```python
from build123d import *

# Parameters (mm, degrees)
SKETCH_1_W             = 220
SKETCH_1_H             = 5.5
EXTRUDE_1_DEPTH        = 5
EXTRUDE_2_DEPTH        = 5
PATTERN_LINEAR_1_COUNT = 35
PATTERN_LINEAR_1_PITCH = 6.283185307
SKETCH_4_W             = 16.5
SKETCH_4_H             = 38
SKETCH_4_R             = 1.25
SKETCH_4_W_2           = 12.5
SKETCH_4_H_2           = 23.5
EXTRUDE_1_2_DEPTH      = 22
SKETCH_5_W             = 12.5
SKETCH_5_H             = 34
CUT_EXTRUDE_1_DEPTH    = 20
SKETCH_6_W             = 9
SKETCH_6_H             = 8
CUT_EXTRUDE_2_DEPTH    = 225.290548174


with BuildPart() as part:
    # 草图1 → Extrude 1 (new body)
    with BuildSketch(Plane.XY):
        with Locations((110, -2.75)):
            Rectangle(SKETCH_1_W, SKETCH_1_H)
    extrude(amount=EXTRUDE_1_DEPTH)

    # 草图2 → 拉伸2 (add)
    with BuildSketch(Plane.XY.offset(5)):
        Polygon((0, 0), (1.637866054, 4.5), (3.323577771, 4.5), (4.961443825, 0), align=None)
    extrude_2 = extrude(amount=-EXTRUDE_2_DEPTH)

    # 阵列(线性)1: 拉伸2 ×35
    with Locations(*[(i * PATTERN_LINEAR_1_PITCH, 0, 0) for i in range(1, PATTERN_LINEAR_1_COUNT)]):
        add(extrude_2)

    # 草图4 → Extrude 1 2 (add)
    with BuildSketch(Plane(origin=(220, 0, 0), x_dir=(0, 0, -1), z_dir=(1, 0, 0))):
        with Locations((-13.25, 13.5)):
            Rectangle(SKETCH_4_W, SKETCH_4_H)
        with Locations((-16.75, 27.5)):
            Circle(SKETCH_4_R, mode=Mode.SUBTRACT)
        with Locations(Location((-9.75, 27.5, 0), (0, 0, 180))):
            Circle(SKETCH_4_R, mode=Mode.SUBTRACT)
        with Locations((-9.75, -0.5)):
            Circle(SKETCH_4_R, mode=Mode.SUBTRACT)
        with Locations(Location((-16.75, -0.5, 0), (0, 0, 180))):
            Circle(SKETCH_4_R, mode=Mode.SUBTRACT)
        with Locations((-13.25, 13.5)):
            Rectangle(SKETCH_4_W_2, SKETCH_4_H_2, mode=Mode.SUBTRACT)
    extrude(amount=-EXTRUDE_1_2_DEPTH)

    # 草图5 → 切除-拉伸1 (cut)
    with BuildSketch(Plane.ZY.offset(-198)):
        with Locations((13.25, 13.5)):
            Rectangle(SKETCH_5_W, SKETCH_5_H)
    extrude(amount=-CUT_EXTRUDE_1_DEPTH, mode=Mode.SUBTRACT)

    # 草图6 → 切除-拉伸2 (cut, through all)
    with BuildSketch(Plane(origin=(0, 32.5, 0), x_dir=(1, 0, 0), z_dir=(0, 1, 0))):
        with Locations((202.5, -13.25)):
            Rectangle(SKETCH_6_W, SKETCH_6_H)
    extrude(amount=-CUT_EXTRUDE_2_DEPTH, mode=Mode.SUBTRACT)


solid = part.part
```
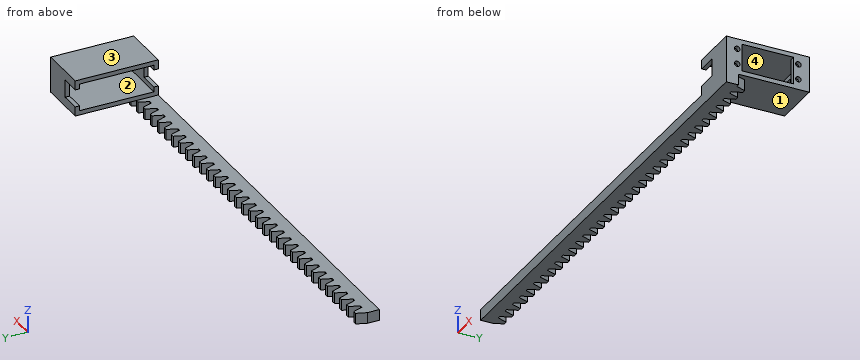
Part model, mm, in its own coordinate system. Face numbers are marked on the shaded views. A direction names the side the tool comes from. Round coordinates to 2 decimals unless told otherwise and drop trailing zeros. Loops run counter-clockwise (first coordinate to the right, second up) from the corner with the lowest first, then second, coordinate; pieces in that order, holes last. Notation, with made-up numbers: (-6, 18) -> (25, 18) arc R22 cw to (25, 26) -> close; hole circle Ø3 at (80.5, 29.25). An arc over 180 degrees is marked (long way). Use one line per item in the form item = value. Start each with the question number.
Item 1: Drill centre lines: line 1 along Y through (x, z) = (218.7, 9.75); line 2 along Z through (x, y) = (209, 21); line 3 along Y through (x, z) = (105.5, 4.75). Where is each one in solid material? Low to high.
Item 2: Drop flat-ended pins along their axis: pin 1 Ø0.8 at (x, z) = (121.5, 1.5) entering from +Y; pin 2 Ø1.6 at (y, z) = (-4.5, 11.5) entering from -X; pin 3 Ø1 at (y, z) = (23.5, 5.5) entering from -X. Give the stop position or say it passes through.
Item 3: Band-saw the part on A-A (y = 17). List the corners of the cut face in (x, z).
Item 4: Two-plate mould, pull along Y, no slides. Class the marked faces 1 and 2: released by +Y, released by -Y, zero draft, split by the parting line, or undercut.
Item 5: Tool access for the marked faces 3 and 4: list every direction of +Z, -Z, +X, -X, +Y, -Y with a clear straight run to the whole face (end or side of a thin tool).
Data:
q1.line_1 = -5.5 to -1.75, 0.75 to 1.75, 25.25 to 26.25, 28.75 to 32.5
q1.line_2 = 5 to 7, 19.5 to 21.5
q1.line_3 = -5.5 to 0
q2.pin_1 = 4.5
q2.pin_2 = 207
q2.pin_3 = 198
q3.outline = (198, 5) -> (220, 5) -> (220, 7) -> (198, 7) -> close; (198, 19.5) -> (220, 19.5) -> (220, 21.5) -> (198, 21.5) -> close
q4.face_1 = zero draft
q4.face_2 = undercut
q5.face_3 = +Z, +X, -X, +Y, -Y
q5.face_4 = -X
